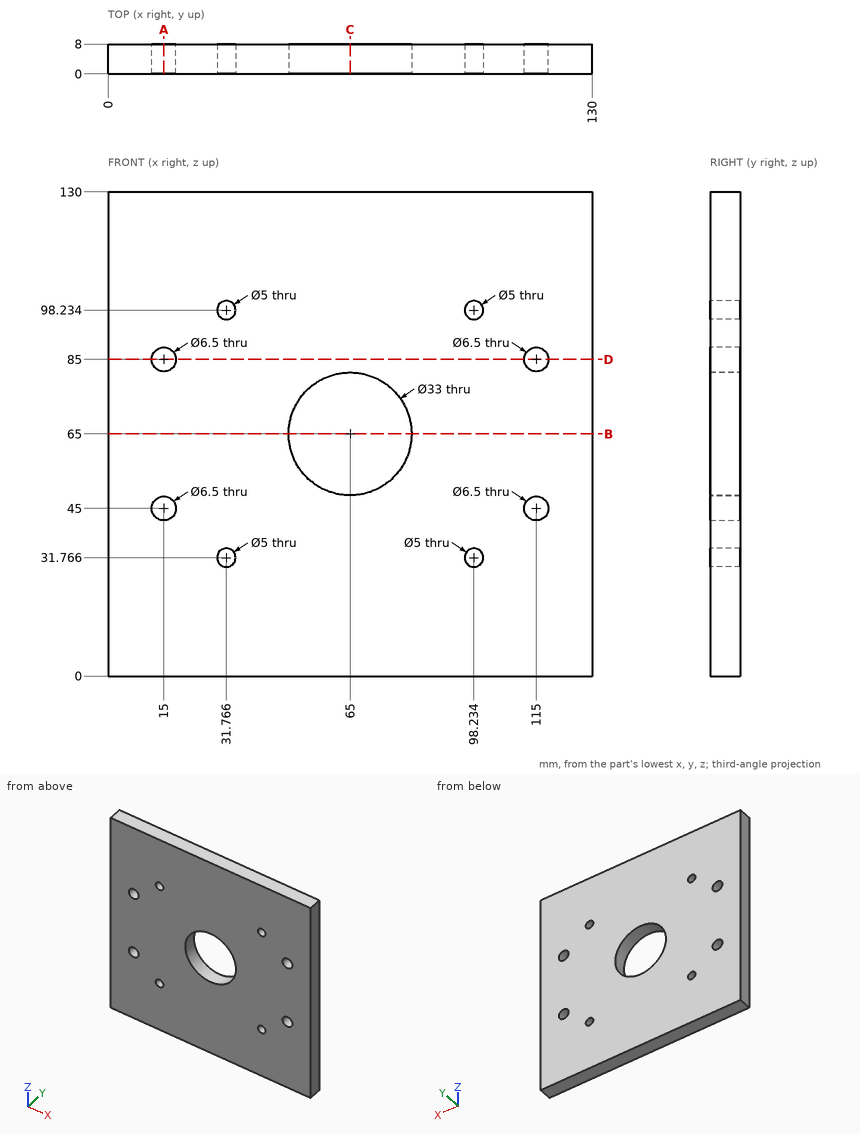
Print and shaded views of the part. All mm, measured from the part's lowest x, y and z. Round coordinates to 2 decimals unless told otherwise and drop trailing zeros. Write each loop counter-clockwise with the first axis right and the second up, starting at its lowest first coordinate (ties: lowest second). Pieces come first, ordered by that corner, then holes. Notation, with made-up numbers: (12, 60) - (57, 60) arc R28 cw to (57, 90) - close; hole circle Ø6 at (-18.5, 58). An arc over 180 degrees is marked (long way). Write each question's results on one line, items separated by ' | '. Start each with the question number.
Item 1: Wall check: L1, parallel to X at y = 2.75, z = 45; L2, parallel to X at y = 4, z = 65; L3, parallel to Z at x = 15, y = 6.25. Give the ranges that are in metal, low to high. Write a range as [from, to].
Item 2: Saw through at D-D (z = 85). Write the cut outline in (x, y).
Item 3: Drop a flat-ended pin along its axis: P1, Ø10.5, axis at x = 15, z = 45, coming from the -Y side. Give the stop position or say it passes through.
Item 4: Saw through at A-A (x = 15). Write the cut outline in (y, z), and give its area (3 significant figures).
Item 5: Saw through at B-B (z = 65). Write the cut outline in (x, y), and give its area (3 significant figures).
Item 6: Saw through at C-C (x = 65). Write the cut outline in (y, z).
Results are:
1) L1: x = [0, 11.75], [18.25, 111.75], [118.25, 130] | L2: x = [0, 48.5], [81.5, 130] | L3: z = [0, 41.75], [48.25, 81.75], [88.25, 130]
2) outline: (0, 0) - (11.75, 0) - (11.75, 8) - (0, 8) - close; (18.25, 0) - (111.75, 0) - (111.75, 8) - (18.25, 8) - close; (118.25, 0) - (130, 0) - (130, 8) - (118.25, 8) - close
3) P1: stops at y = 0
4) outline: (0, 0) - (8, 0) - (8, 41.75) - (0, 41.75) - close; (0, 48.25) - (8, 48.25) - (8, 81.75) - (0, 81.75) - close; (0, 88.25) - (8, 88.25) - (8, 130) - (0, 130) - close | area: 936 mm²
5) outline: (0, 0) - (48.5, 0) - (48.5, 8) - (0, 8) - close; (81.5, 0) - (130, 0) - (130, 8) - (81.5, 8) - close | area: 776 mm²
6) outline: (0, 0) - (8, 0) - (8, 48.5) - (0, 48.5) - close; (0, 81.5) - (8, 81.5) - (8, 130) - (0, 130) - close
